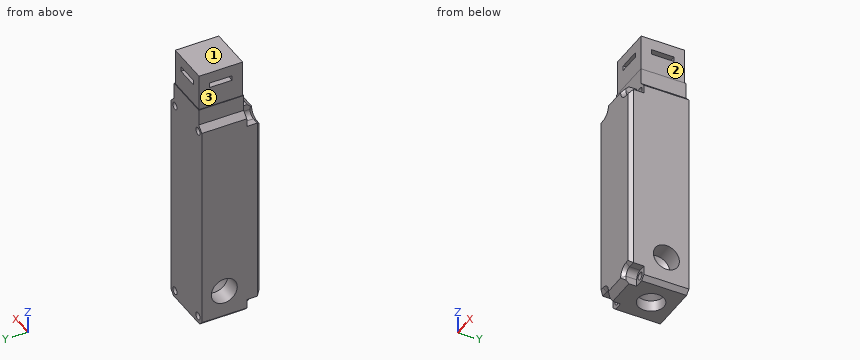
from build123d import *

# Parameters (mm, degrees)
SKIZZE1_R                       = 2.65
AUFSATZ_LINEAR_AUSTRAGEN1_DEPTH = 32
SKIZZE2_W                       = 31
SKIZZE2_H                       = 31
AUFSATZ_LINEAR_AUSTRAGEN2_DEPTH = 26
AUFSATZ_LINEAR_AUSTRAGEN3_DEPTH = 10
FASE2_SIZE                      = 4.5
FASE1_SIZE                      = 2.5
M20X1_5_GEWINDEBOHRUNG1_D       = 18.5
M20X1_5_GEWINDEBOHRUNG1_DEPTH   = 8
M20X1_5_GEWINDEBOHRUNG1_TIP     = 5.557960726
M20X1_5_GEWINDEBOHRUNG2_D       = 18.5
M20X1_5_GEWINDEBOHRUNG2_DEPTH   = 12.5
M20X1_5_GEWINDEBOHRUNG2_TIP     = 5.557960726
M20X1_5_GEWINDEBOHRUNG3_D       = 18.5
M20X1_5_GEWINDEBOHRUNG3_DEPTH   = 12.5
M20X1_5_GEWINDEBOHRUNG3_TIP     = 5.557960726
SKIZZE10_W                      = 6
SKIZZE10_H                      = 16
SKIZZE10_W_2                    = 16
SKIZZE10_H_2                    = 6
SCHNITT_LINEAR_AUSTRAGEN1_DEPTH = 3.5


with BuildPart() as part:
    # Skizze1 → Aufsatz-Linear austragen1 (new body)
    with BuildSketch(Plane(origin=(0, 0, 0), x_dir=(1, 0, 0), z_dir=(0, 1, 0))):
        Polygon((16, -17), (-16, -17), (-16, -5.5), (-20, -1.5), (-20, 146), (-17, 149), (17, 149), (20, 146), (20, -1.5), (16, -5.5), align=None)
        with Locations(Location((15, 0, 0), (0, 0, 270))):
            Circle(SKIZZE1_R, mode=Mode.SUBTRACT)
        with Locations(Location((-15, 0, 0), (0, 0, 270))):
            Circle(SKIZZE1_R, mode=Mode.SUBTRACT)
        with Locations(Location((-15, 144, 0), (0, 0, 270))):
            Circle(SKIZZE1_R, mode=Mode.SUBTRACT)
        with Locations(Location((15, 144, 0), (0, 0, 270))):
            Circle(SKIZZE1_R, mode=Mode.SUBTRACT)
    extrude(amount=-AUFSATZ_LINEAR_AUSTRAGEN1_DEPTH)

    # Skizze2 → Aufsatz-Linear austragen2 (add)
    with BuildSketch(Plane.XY.offset(17)):
        with Locations((0, -16)):
            Rectangle(SKIZZE2_W, SKIZZE2_H)
    extrude(amount=AUFSATZ_LINEAR_AUSTRAGEN2_DEPTH)

    # Skizze3 → Aufsatz-Linear austragen3 (add)
    with BuildSketch(Plane.XZ.offset(32)):
        with BuildLine():
            Line((20, -4.5), (15, -4.5))
            ThreePointArc((15, -4.5), (11.818019485, -3.181980515), (10.5, 0))
            Line((10.5, 0), (10.5, 4.5))
            Line((10.5, 4.5), (-10.5, 4.5))
            Line((-10.5, 4.5), (-10.5, 0))
            ThreePointArc((-10.5, 0), (-11.818019485, -3.181980515), (-15, -4.5))
            Line((-15, -4.5), (-20, -4.5))
            Line((-20, -4.5), (-20, -139.5))
            Line((-20, -139.5), (-15, -139.5))
            ThreePointArc((-15, -139.5), (-11.818019485, -140.818019485), (-10.5, -144))
            Line((-10.5, -144), (-10.5, -149))
            Line((-10.5, -149), (10.5, -149))
            Line((10.5, -149), (10.5, -144))
            ThreePointArc((10.5, -144), (11.818019485, -140.818019485), (15, -139.5))
            Line((15, -139.5), (20, -139.5))
            Line((20, -139.5), (20, -4.5))
        make_face()
    extrude(amount=AUFSATZ_LINEAR_AUSTRAGEN3_DEPTH)

    # Fase2
    fase2_edges = [part.edges().sort_by_distance(p)[0] for p in [
        (0, -42, 4.5),
        (0, -42, -149),
    ]]
    chamfer(fase2_edges, length=FASE2_SIZE)

    # Fase1
    # the kernel refuses this chamfer: 2.5 mm, written as the material it takes off along each edge
    with BuildSketch(Plane(origin=(10.5, -42, -150.92920747), x_dir=(0.027495876610586282, 0.9996219169112968, 0), z_dir=(0, 0, 1)), Plane(origin=(-10.5, -42, -144), x_dir=(-0.027495876610586282, 0.9996219169112968, 0), z_dir=(0, 0, -1))) as fase1_piece_1:
        Polygon((FASE1_SIZE * 0.999621916911, FASE1_SIZE * 0.0274958766106), (-FASE1_SIZE * 0.0274958766106, FASE1_SIZE * 0.999621916911), (0, 0), align=None)
    extrude(amount=6.92920747, mode=Mode.SUBTRACT)
    with BuildSketch(Plane(origin=(20, -42, -145.92920747), x_dir=(-0.9996219169112968, -0.0274958766105877, 0), z_dir=(0, 0, 1)), Plane(origin=(-20, -42, 1.92920747), x_dir=(0.9996219169112968, -0.0274958766105877, 0), z_dir=(0, 0, -1))) as fase1_piece_2:
        Polygon((FASE1_SIZE * 0.999621916911, -FASE1_SIZE * 0.0274958766106), (-FASE1_SIZE * 0.0274958766106, -FASE1_SIZE * 0.999621916911), (0, 0), align=None)
    extrude(amount=147.85841494, mode=Mode.SUBTRACT)
    with BuildSketch(Plane(origin=(26.42920747, -42, -4.5), x_dir=(0, -0.0274958766105877, -0.9996219169112968), z_dir=(-1, 0, 0)), Plane(origin=(-15, -42, -4.5), x_dir=(0, -0.0274958766105877, -0.9996219169112968), z_dir=(-1, 0, 0)), Plane(origin=(-26.42920747, -42, -139.5), x_dir=(0, -0.027495876610587815, 0.9996219169112968), z_dir=(1, 0, 0)), Plane(origin=(15, -42, -139.5), x_dir=(0, -0.027495876610587815, 0.9996219169112968), z_dir=(1, 0, 0))) as fase1_piece_3:
        Polygon((FASE1_SIZE * 0.999621916911, -FASE1_SIZE * 0.0274958766106), (-FASE1_SIZE * 0.0274958766106, -FASE1_SIZE * 0.999621916911), (0, 0), align=None)
    extrude(amount=11.42920747, mode=Mode.SUBTRACT)
    with BuildSketch(Plane(origin=(15, -42, 0), x_dir=(0, 0, -1), z_dir=(1, 0, 0))) as fase1_piece_4:
        Polygon((4.5 + FASE1_SIZE, 0), (4.5, FASE1_SIZE), (4.5, 0), align=None)
    revolve(axis=Axis((15, -42, 0), (0, 1, 0)), revolution_arc=171.892095433, mode=Mode.SUBTRACT)
    with BuildSketch(Plane(origin=(-15, -42, 0), x_dir=(0.14103781497281773, 0, 0.9900042094595827), z_dir=(-0.9900042094595827, 0, 0.14103781497281773))) as fase1_piece_5:
        Polygon((4.5 + FASE1_SIZE, 0), (4.5, FASE1_SIZE), (4.5, 0), align=None)
    revolve(axis=Axis((-15, -42, 0), (0, 1, 0)), revolution_arc=171.892095433, mode=Mode.SUBTRACT)
    with BuildSketch(Plane(origin=(-15, -42, -144), x_dir=(0, 0, 1), z_dir=(-1, 0, 0))) as fase1_piece_6:
        Polygon((4.5 + FASE1_SIZE, 0), (4.5, FASE1_SIZE), (4.5, 0), align=None)
    revolve(axis=Axis((-15, -42, -144), (0, 1, 0)), revolution_arc=90, mode=Mode.SUBTRACT)
    with BuildSketch(Plane(origin=(15, -42, -144), x_dir=(-1, 0, 0), z_dir=(0, 0, -1))) as fase1_piece_7:
        Polygon((4.5 + FASE1_SIZE, 0), (4.5, FASE1_SIZE), (4.5, 0), align=None)
    revolve(axis=Axis((15, -42, -144), (0, 1, 0)), revolution_arc=90, mode=Mode.SUBTRACT)

    # M20x1.5 Gewindebohrung1
    with Locations(Plane(origin=(0, 0, -149), x_dir=(-1, 0, 0), z_dir=(0, 0, -1))):
        with Locations((0, -16)):
            Hole(M20X1_5_GEWINDEBOHRUNG1_D / 2, depth=M20X1_5_GEWINDEBOHRUNG1_DEPTH)
            with Locations((0, 0, -(M20X1_5_GEWINDEBOHRUNG1_DEPTH + M20X1_5_GEWINDEBOHRUNG1_TIP / 2))):  # 118° drill point
                Cone(0, M20X1_5_GEWINDEBOHRUNG1_D / 2, M20X1_5_GEWINDEBOHRUNG1_TIP, mode=Mode.SUBTRACT)

    # M20x1.5 Gewindebohrung2
    with Locations(Plane.ZY.offset(20)):
        with Locations((-127, -16)):
            Hole(M20X1_5_GEWINDEBOHRUNG2_D / 2, depth=M20X1_5_GEWINDEBOHRUNG2_DEPTH)
            with Locations((0, 0, -(M20X1_5_GEWINDEBOHRUNG2_DEPTH + M20X1_5_GEWINDEBOHRUNG2_TIP / 2))):  # 118° drill point
                Cone(0, M20X1_5_GEWINDEBOHRUNG2_D / 2, M20X1_5_GEWINDEBOHRUNG2_TIP, mode=Mode.SUBTRACT)

    # M20x1.5 Gewindebohrung3
    with Locations(Plane(origin=(20, 0, 0), x_dir=(0, 0, -1), z_dir=(1, 0, 0))):
        with Locations((127, -16)):
            Hole(M20X1_5_GEWINDEBOHRUNG3_D / 2, depth=M20X1_5_GEWINDEBOHRUNG3_DEPTH)
            with Locations((0, 0, -(M20X1_5_GEWINDEBOHRUNG3_DEPTH + M20X1_5_GEWINDEBOHRUNG3_TIP / 2))):  # 118° drill point
                Cone(0, M20X1_5_GEWINDEBOHRUNG3_D / 2, M20X1_5_GEWINDEBOHRUNG3_TIP, mode=Mode.SUBTRACT)

    # Skizze10 → Schnitt-Linear austragen1 (cut)
    with BuildSketch(Plane.XY.offset(35)):
        with Locations((12.5, -16)):
            Rectangle(SKIZZE10_W, SKIZZE10_H)
        with Locations((0, -28.5)):
            Rectangle(SKIZZE10_W_2, SKIZZE10_H_2)
        with Locations((-12.5, -16)):
            Rectangle(SKIZZE10_W, SKIZZE10_H)
        with Locations((0, -3.5)):
            Rectangle(SKIZZE10_W_2, SKIZZE10_H_2)
    extrude(amount=-SCHNITT_LINEAR_AUSTRAGEN1_DEPTH, mode=Mode.SUBTRACT)


solid = part.part
For this review, take the finished solid that the model builds, in its own axes (mm). Face numbers are marked on the shaded views. A direction names the side the tool comes from. Give positions to 0.01 mm unless a question says otherwise; leave off trailing zeros. Order: outer loops, then holes, each group sorted by start corner. A loop starts at its lowest first (then second) coordinate and runs counter-clockwise, first axis right, second up. Notation, with made-up numbers: M 33,32.25 L 88,32.25 A31 ccw 88,67.25 Z; hole C 11.5,31.5 d4. An arc over 180 degrees is marked long. Answer in a Markdown table with one row per item. Add a question column.
(1) For the marked faces 1, 2 and 3, list the 3-axis set-ups (+Z, -Z, +X, -X, +Y, -Y) from which the entire face can be reached by the end or side of a thin tool; tool diameter is ignored.
(2) Consider section B-B on y = -10.5. Give the number of separate pieces and of enclosed holes in the cut face, and give its area (3 significant figures).
(3) Wall thickness on probe 1 along X at (y, z) = (-9.5, 0); probe 2 along Y at (x, z) = (10, -127); probe 3 along Z at (x, y) = (10, -12.5): over which ranges is each line inside the solid? List them lowest first. Write a range as [from, to].
(4) Consider section A-A on y = -35. State the section outline as (x, z) points.
(5) For pin 1 (8 mm diameter, centred on x = 2.5, z = -11, fed in from +Y); pin 2 (8.5 mm diameter, centred on x = -15, z = 0, fed in from -Y); pin 3 (1.5 mm diameter, centred on y = -35, z = -147, fed in from +X); pin 4 (4 mm diameter, centred on y = -34.5, z = -145.5, fed in from -X), all flat-tipped, find the tip position at first contact; note any pin that passes through.
Evaluation:
| question | item | result |
|---|---|---|
| 1 | face 1 | +Z, +X, -X, +Y, -Y |
| 1 | face 2 | +Z, +X, +Y, -Y |
| 1 | face 3 | +Z, -X, +Y, -Y |
| 2 | separate pieces | 1 |
| 2 | enclosed holes | 4 |
| 2 | area | 6,640 mm^2 |
| 3 | probe 1 | x = [-20, -17.65], [-12.35, 12.35], [17.65, 20] |
| 3 | probe 2 | y = [-42, -25.25], [-6.75, 0] |
| 3 | probe 3 | z = [-149, -135.56], [-118.44, 31.5], [35, 43] |
| 4 | outline | M -20,-139.5 L -15,-139.5 A4.5 cw -10.5,-144 L -10.5,-149 L 10.5,-149 L 10.5,-144 A4.5 cw 15,-139.5 L 20,-139.5 L 20,-4.5 L 15,-4.5 A4.5 cw 10.5,0 L 10.5,4.5 L -10.5,4.5 L -10.5,0 A4.5 cw -15,-4.5 L -20,-4.5 Z |
| 5 | pin 1 | stops at y = 0 |
| 5 | pin 2 | stops at y = -32 |
| 5 | pin 3 | stops at x = 10.5 |
| 5 | pin 4 | stops at x = -10.53 |
